Solid Edge part; units mm, degrees
sketch "Sketch1" plane through (0, 0, 0) normal (0, 0, 1) x (1, 0, 0)
  line L0 (120, 40) -> (0, 40)
  line L1 (0, 40) -> (0, 0)
  line L2 (0, 0) -> (120, 0)
  line L3 (120, 0) -> (120, 40)
extrude "Protrusion1" add sketch "Sketch1" along normal blind 5
sketch "Sketch2" plane through (60, 20, 5) normal (0, 0, 1) x (1, 0, 0)
  line L0 (55, -20) -> (55, 20)
  line L1 (55, 20) -> (60, 20)
  line L2 (60, 20) -> (60, -20)
  line L3 (60, -20) -> (55, -20)
  line L4 (-55, 20) -> (-55, -20)
  line L5 (-55, -20) -> (-60, -20)
  line L6 (-60, -20) -> (-60, 20)
  line L7 (-60, 20) -> (-55, 20)
extrude "Extrusionsausprägung_2" add sketch "Sketch2" along normal blind 60
hole "Bohrung_1" at (120, 20, 45) direction (-1, 0, 0) diameter 10 end up to next
hole "Hole_2" at (20, 10, 5) direction (0, 0, -1) diameter 4.2 end up to next start chamfer 0.6 start chamfer angle 45
hole "Hole1" at (20, 30, 5) direction (0, 0, -1) diameter 4.2 end up to next start chamfer 0.6 start chamfer angle 45
hole "Hole2" at (100, 30, 5) direction (0, 0, -1) diameter 4.2 end up to next start chamfer 0.6 start chamfer angle 45
hole "Hole3" at (100, 10, 5) direction (0, 0, -1) diameter 4.2 end up to next start chamfer 0.6 start chamfer angle 45
hole "Hole4" at (120, 9, 56) direction (-1, 0, 0) diameter 4.2 end up to next
hole "Hole5" at (120, 9, 34) direction (-1, 0, 0) diameter 4.2 end up to next
hole "Hole6" at (120, 31, 34) direction (-1, 0, 0) diameter 4.2 end up to next
hole "Hole7" at (120, 31, 56) direction (-1, 0, 0) diameter 4.2 end up to next
hole "Hole_10" at (0, 20, 45) direction (1, 0, 0) diameter 8 end up to next
Verification items for the finished model (mm, model axes). A direction names the side the tool comes from. Coordinates: 2 decimals unless noted, no trailing zeros. Order: outer loops, then holes, each group sorted by start corner. A loop starts at its lowest first (then second) coordinate and runs counter-clockwise, first axis right, second up. Notation, with made-up numbers: M 57,41.5 L 96,41.5 A30 ccw 96,66.5 Z; hole C -4,21 d11. An arc over 180 degrees is marked long. Write each question's results on one line, items separated by ' | '.
1) Scan lines: line 1 along Z through (x, y) = (116, 31); line 2 along Y through (x, z) = (118.8, 56); line 3 along Y through (x, z) = (20, 3.35). Record each from-to range of solid material in increasing order. Write a range as [from, to].
Solved:
line 1: z = [0, 31.9], [36.1, 53.9], [58.1, 65] | line 2: y = [0, 6.9], [11.1, 28.9], [33.1, 40] | line 3: y = [0, 7.9], [12.1, 27.9], [32.1, 40]
2) Release check for a two-part mould opening along X. For faces 4 (the face through (3, 20, 65)), 5 (the face through (0, 20, 32)), 6 (the face through (115, 20, 35)) record: pulls with the +X half, pulls with the -X half, needs draft (parallel to the pull), parting line crosses it, or undercut.
Solved:
face 4: needs draft | face 5: pulls with the -X half | face 6: undercut
3) Section check C-C on z = 13. Record the cut outline in (x, y).
Solved:
outline: M 0,0 L 5,0 L 5,40 L 0,40 Z; M 115,0 L 120,0 L 120,40 L 115,40 Z
4) Section check D-D on x = 68.5. Record the cut outline in (y, z), plus the area to 3 significant figures.
Solved:
outline: M 0,0 L 40,0 L 40,5 L 0,5 Z | area: 200 mm²
5) Section check B-B on x = 20. Record the cut outline in (y, z), plus the area to 3 significant figures.
Solved:
outline: M 0,0 L 7.9,0 L 7.9,4.4 L 7.3,5 L 0,5 Z; M 12.1,0 L 27.9,0 L 27.9,4.4 L 27.3,5 L 12.7,5 L 12.1,4.4 Z; M 32.1,0 L 40,0 L 40,5 L 32.7,5 L 32.1,4.4 Z | area: 157 mm²
6) Access from +Z, -Z, +X, -X, +Y, -Y to the whole of each face (thin tool, end or side, straight path). Record for faces 1 (the face through (118, 20, 65)), 2 (the face through (117.54, 9.09, 36.1)), 3 (the face through (59, 20, 5)).
Solved:
face 1: +Z, +X, -X, +Y, -Y | face 2: +X | face 3: +Z, +Y, -Y
7) Gauge pin test, flat ends, axial feed: pin 1 Ø5 at (x, y) = (20, 10) entering from +Z; pin 2 Ø10 at (x, y) = (17.5, 27) entering from +Z. Record the tip position at first contact, or that the pin passes through.
Solved:
pin 1: stops at z = 4.8 | pin 2: stops at z = 5
8) Section check A-A on z = 45. Record the cut outline in (x, y).
Solved:
outline: M 0,0 L 5,0 L 5,16 L 0,16 Z; M 0,24 L 5,24 L 5,40 L 0,40 Z; M 115,0 L 120,0 L 120,15 L 115,15 Z; M 115,25 L 120,25 L 120,40 L 115,40 Z
